Build history of the part. All positions in model axes, mm. A direction names the side the tool comes from. Round coordinates to 2 decimals unless told otherwise and drop trailing zeros. Order: outer loops, then holes, each group sorted by start corner. A loop starts at its lowest first (then second) coordinate and runs counter-clockwise, first axis right, second up. Notation, with made-up numbers: M 45.25,8 L 73.25,8 A19 cw 73.25,24 Z; hole C 1,-3 d3. An arc over 180 degrees is marked long. One line per question, with ' | ' between items. Start each with the question number.
from build123d import *

# Parameters (mm, degrees)
F1_DEPTH = 15.24
F2_T     = -2.54
F3_R     = 5.08
F5_D     = 18.47
F5_DEPTH = 14
F5_TIP   = 5.5489478167


with BuildPart() as f1:
    # F0 (on Front) → F1 (new body)
    with BuildSketch(Plane.XZ):
        Polygon((86.5705514472, 17.0364904519), (86.5705514472, 57.0414904519), (-110.0254485528, 57.0414904519), (-110.0254485528, -84.2587095481), (-47.6176485528, -84.2587095481), (-47.6176485528, 17.0364904519), align=None)
    extrude(amount=F1_DEPTH)

    # F2
    f2_openings = [f1.faces().sort_by_distance(p)[0] for p in [
        (19.476451, 0, 19.457559),
    ]]
    offset(amount=F2_T, openings=f2_openings, kind=Kind.INTERSECTION)

    # F3
    f3_edges = [f1.edges().sort_by_distance(p)[0] for p in [
        (-110.025449, -15.24, -13.60861),
        (-47.617649, -15.24, -33.61111),
        (-78.821549, -15.24, -84.25871),
        (-110.025449, -7.62, -84.25871),
        (-11.727449, -15.24, 57.04149),
        (19.476451, -15.24, 17.03649),
        (-110.025449, -7.62, 57.04149),
        (86.570551, -15.24, 37.03899),
        (86.570551, -7.62, 57.04149),
        (86.570551, -7.62, 17.03649),
        (-47.617649, -7.62, -84.25871),
    ]]
    fillet(f3_edges, radius=F3_R)

    # F5
    with Locations(Plane.YZ.offset(86.5705514472)):
        with Locations((0, 37.0389904519)):
            Hole(F5_D / 2, depth=F5_DEPTH)
            with Locations((0, 0, -(F5_DEPTH + F5_TIP / 2))):  # 118° drill point
                Cone(0, F5_D / 2, F5_TIP, mode=Mode.SUBTRACT)


solid = f1.part
Item 1: Two-plate mould, pull along Z, no slides. Class faces 5 (the face through (-50.158, -6, -32)), 6 (the face through (-79, -5, -84.259)), 7 (the face through (-108.5, -5.15, 55.59)): +Z half, -Z half, draft (parallel to the pull), parting line (faces both ways), or undercut.
Item 2: Cut at C-C on y = -7. Write the cut outline in (x, z).
Item 3: Cut at A-A on z = -12. Write the cut outline in (x, y).
Item 4: Wall check: line 1 along X through (y, z) = (-1.75, -31); line 2 along Z through (x, y) = (-31.5, -9.5); line 3 along Z through (x, y) = (-74, -10). Give the ranges that are in metal, low to high. Write a range as [from, to].
Item 5: Cut at B-B on x = 34.5. Write the cut outline in (y, z), then the cut area to 3 significant figures.
Item 6: Tool access for faces 1 (the face through (85.283, -9.233, 36.836)), 2 (the face through (15.336, -13.712, 18.485)), 3 (the face through (-107.485, -6, -13)), 4 (the face through (-47.618, -5, -32)): list every direction of +Z, -Z, +X, -X, +Y, -Y with a clear straight run to the whole face (end or side of a thin tool).
Item 7: Flat gauge pins, fed straight in: pin 1 (8 mm diameter, centred on x = 35.5, y = -4, fed in from -Z); pin 2 (6.5 mm diameter, centred on y = -6, z = -10.5, fed in from +X). Where does each tip first touch, or does it go through?
Results found:
1) face 5: undercut | face 6: -Z half | face 7: +Z half
2) outline: M -110.03,-79.18 A5.08 ccw -104.95,-84.26 L -52.7,-84.26 A5.08 ccw -47.62,-79.18 L -47.62,17.04 L 81.49,17.04 A5.08 ccw 86.57,22.12 L 86.57,31.02 L 84.03,31.02 L 84.03,19.58 L -50.16,19.58 L -50.16,-81.72 L -107.49,-81.72 L -107.49,54.5 L 84.03,54.5 L 84.03,43.06 L 86.57,43.06 L 86.57,51.96 A5.08 ccw 81.49,57.04 L -104.95,57.04 A5.08 ccw -110.03,51.96 Z
3) outline: M -110.03,-10.16 A5.08 ccw -104.95,-15.24 L -52.7,-15.24 A5.08 ccw -47.62,-10.16 L -47.62,0 L -50.16,0 L -50.16,-12.7 L -107.49,-12.7 L -107.49,0 L -110.03,0 Z
4) line 1: x = [-110.03, -107.49], [-50.16, -47.62] | line 2: z = [17.04, 19.58], [54.5, 57.04] | line 3: z = [-84.26, -81.72], [54.5, 57.04]
5) outline: M -15.24,22.12 A5.08 ccw -10.16,17.04 L 0,17.04 L 0,19.58 L -12.7,19.58 L -12.7,54.5 L 0,54.5 L 0,57.04 L -10.16,57.04 A5.08 ccw -15.24,51.96 Z | area: 155 mm^2
6) face 1: +X, +Y | face 2: -Z, +X, -Y | face 3: +Y | face 4: -Z, +X, +Y, -Y
7) pin 1: stops at z = 17.04 | pin 2: stops at x = -47.62
